The figure shows three views and two pictorial views of one solid part (mm, origin at its lowest corner). Answer the questions. A direction names the side the tool comes from. Coordinates: 2 decimals unless noted, no trailing zeros. Order: outer loops, then holes, each group sorted by start corner. A loop starts at its lowest first (then second) coordinate and runs counter-clockwise, first axis right, second up. Notation, with made-up numbers: (-24, 82.25) -> (19, 82.25) arc R24 ccw to (19, 110.25) -> close; hole circle Ø1 at (-13.5, -15.75). An arc over 180 degrees is marked (long way). Write item = value, one per line. Start each with the question number.
Q1. The part is cut by section C-C, the plane x = 47.5. Determine the outline of the cut face in (y, z), plus the area to 3 significant figures.
Q2. Straight lines are drawn through the part: L1, parallel to Z at x = 22, y = 34; L2, parallel to X at y = 22, z = 2.5. For each, find the intervals that lie inside material, in ascending order. Write a range as from..to.
Q3. The part is cut by section A-A, the plane y = 6. Determine the outline of the cut face in (x, z), plus the area to 3 significant figures.
Q4. Which of the six approach directions +Z, -Z, +X, -X, +Y, -Y give full straight-line access (tool end or side, diameter ignored) to the marked faces 1, 2 and 3?
Q5. The part is cut by section B-B, the plane z = 16. Determine the outline of the cut face in (x, y), plus the area to 3 significant figures.
Q6. The part is cut by section D-D, the plane y = 22.5. Determine the outline of the cut face in (x, z).
Q7. Flat-ended cylindrical pins translate along their axes: pin 1 (9.5 mm diameter, centred on x = 12, z = 10, fed in from +Y); pin 2 (15 mm diameter, centred on y = 31.5, z = 6, fed in from -X); pin 3 (15 mm diameter, centred on y = 11.5, z = 30, fed in from +X). Find the tip coordinate at first contact, or state that the pin passes through.
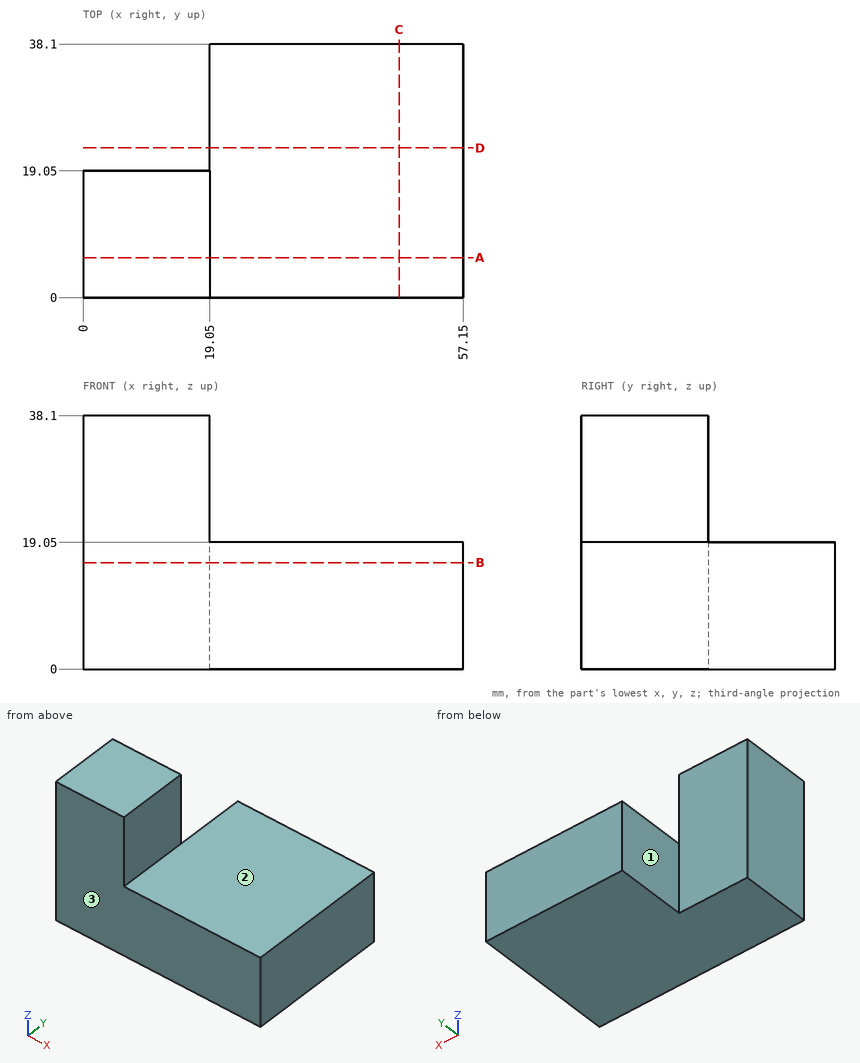
Model answer:
q1.outline = (0, 0) -> (38.1, 0) -> (38.1, 19.05) -> (0, 19.05) -> close
q1.area = 726 mm2
q2.L1 = 0..19.05
q2.L2 = 19.05..57.15
q3.outline = (0, 0) -> (57.15, 0) -> (57.15, 19.05) -> (19.05, 19.05) -> (19.05, 38.1) -> (0, 38.1) -> close
q3.area = 1,450 mm2
q4.face_1 = +Z, -Z, -X, +Y
q4.face_2 = +Z, +X, +Y, -Y
q4.face_3 = +Z, -Z, +X, -X, -Y
q5.outline = (0, 0) -> (57.15, 0) -> (57.15, 38.1) -> (19.05, 38.1) -> (19.05, 19.05) -> (0, 19.05) -> close
q5.area = 1,810 mm2
q6.outline = (19.05, 0) -> (57.15, 0) -> (57.15, 19.05) -> (19.05, 19.05) -> close
q7.pin_1 = 19.05
q7.pin_2 = 19.05
q7.pin_3 = 19.05
